The listing builds one solid part. Answer for the finished solid, in the listing's coordinates (mm). A direction names the side the tool comes from. Coordinates: 2 decimals unless noted, no trailing zeros. Order: outer loops, then holes, each group sorted by start corner. A loop starts at its lowest first (then second) coordinate and runs counter-clockwise, first axis right, second up.
```python
from build123d import *

# Parameters (mm, degrees)
EXTRUDE_THIN1_DEPTH = 539.75
FILLET1_R           = 1.27


with BuildPart() as part:
    # Sketch1 → Extrude-Thin1 (new body)
    with BuildSketch(Plane.XY):
        with BuildLine():
            Line((0, 0), (-4.7625, 0))
            Line((-4.7625, 0), (-4.7625, 2.38125))
            ThreePointArc((-4.7625, 2.38125), (-9.892743248, 5.471846434), (-11.90625, 11.1125))
            Line((-11.90625, 11.1125), (-15.875, 11.1125))
            Line((-15.875, 11.1125), (-15.875, 30.1625))
            Line((-15.875, 30.1625), (-19.05, 30.1625))
            Line((-19.05, 30.1625), (-17.682307692, 35.547788462))
            ThreePointArc((-17.682307692, 35.547788462), (-18.967315097, 41.692088258), (-24.60625, 44.45))
            Line((-24.60625, 44.45), (-26.19375, 53.975))
            ThreePointArc((-26.19375, 53.975), (-19.37999398, 52.288155979), (-14.140184362, 47.617277151))
            Line((-14.140184362, 47.617277151), (-12.847315638, 45.727722849))
            ThreePointArc((-12.847315638, 45.727722849), (-7.60750602, 41.056844021), (-0.79375, 39.37))
            Line((-0.79375, 39.37), (-0.79375, 38.1))
            ThreePointArc((-0.79375, 38.1), (-8.200006544, 39.93352611), (-13.89545178, 45.010568314))
            Line((-13.89545178, 45.010568314), (-15.188320504, 46.900122616))
            ThreePointArc((-15.188320504, 46.900122616), (-19.312101481, 50.792133717), (-24.680202995, 52.618826381))
            Line((-24.680202995, 52.618826381), (-23.518633198, 45.649407601))
            ThreePointArc((-23.518633198, 45.649407601), (-17.64421442, 42.030786976), (-16.451384615, 35.235173077))
            Line((-16.451384615, 35.235173077), (-17.417142857, 31.4325))
            Line((-17.417142857, 31.4325), (-14.605, 31.4325))
            Line((-14.605, 31.4325), (-14.605, 12.3825))
            Line((-14.605, 12.3825), (-10.529920944, 12.3825))
            ThreePointArc((-10.529920944, 12.3825), (-8.987461499, 6.372542318), (-3.4925, 3.490846534))
            Line((-3.4925, 3.490846534), (-3.4925, 1.27))
            Line((-3.4925, 1.27), (0, 1.27))
            Line((0, 1.27), (0, 0))
        make_face()
    extrude(amount=-EXTRUDE_THIN1_DEPTH)

    # Fillet1
    fillet1_edges = [part.edges().sort_by_distance(p)[0] for p in [
        (-14.605, 31.4325, -269.875),
        (-10.529920944, 12.3825, -269.875),
        (-3.4925, 3.490846534, -269.875),
        (-4.7625, 0, -269.875),
        (-15.875, 11.1125, -269.875),
        (-19.05, 30.1625, -269.875),
        (-24.60625, 44.45, -269.875),
        (-26.19375, 53.975, -269.875),
    ]]
    fillet(fillet1_edges, radius=FILLET1_R)


solid = part.part
```
(1) Each of these flat-tipped pins is pushed along its axis until it touches: pin 1 Ø6 at (y, z) = (21, -446.5) entering from -X (3 decimals); pin 2 Ø0.5 at (x, z) = (-17, -395.5) entering from +Y; pin 3 Ø3 at (x, z) = (-13.5, -404.5) entering from +Y. Where does it stop, or does it pass through?
(2) For faces 5 (the face through (-18.732, 51.925, -266.097)), 6 (the face through (-14.605, 21, -266)), 7 (the face through (-18.65, 41.25, -266.1)), 8 (the face through (-17.7, 42.11, -266.1)), 9 (the face through (-15.875, 21, -266)), determine the directions among +Z, -Z, +X, -X, +Y, -Y from which every point of the face is accessible in a straight line to the end or side of a thin tool.
(3) The mould has two halves that part along Y. Classify faces 1 (the face through (-8.1, 39.88, -266.1)), 2 (the face through (-9.84, 5.41, -266.1)), 3 (the face through (-7.695, 41.103, -266.097)), 4 (the face through (-16, 31, -539.75)): released by +Y, released by -Y, zero draft, split by the parting line, or undercut.
(4) Find section B-B (y = 19). Write down the section's boundary in (x, z) (3 decimals).
(5) Consider line 1 (X direction, y = 38, z = -125); line 2 (X direction, y = 28.5, z = -445.5) (3 decimals); line 3 (Y direction, x = -21.75, z = -411). Determine where each line is inside the solid, lowest interval first.
Findings below:
1. pin 1: stops at x = -15.875
1. pin 2: stops at y = 50.92
1. pin 3: stops at y = 48.75
2. face 5: +Z, -Z, +X, +Y
2. face 6: +Z, -Z, +X
2. face 7: +Z, -Z, -X
2. face 8: +Z, -Z
2. face 9: +Z, -Z, -X, -Y
3. face 1: undercut
3. face 2: released by -Y
3. face 3: released by +Y
3. face 4: zero draft
4. outline: (-15.875, -539.75) - (-14.605, -539.75) - (-14.605, 0) - (-15.875, 0) - close
5. line 1: x = -17.5 to -16.22
5. line 2: x = -15.875 to -14.605
5. line 3: y = 43.85 to 45.22, 51.94 to 53.28
